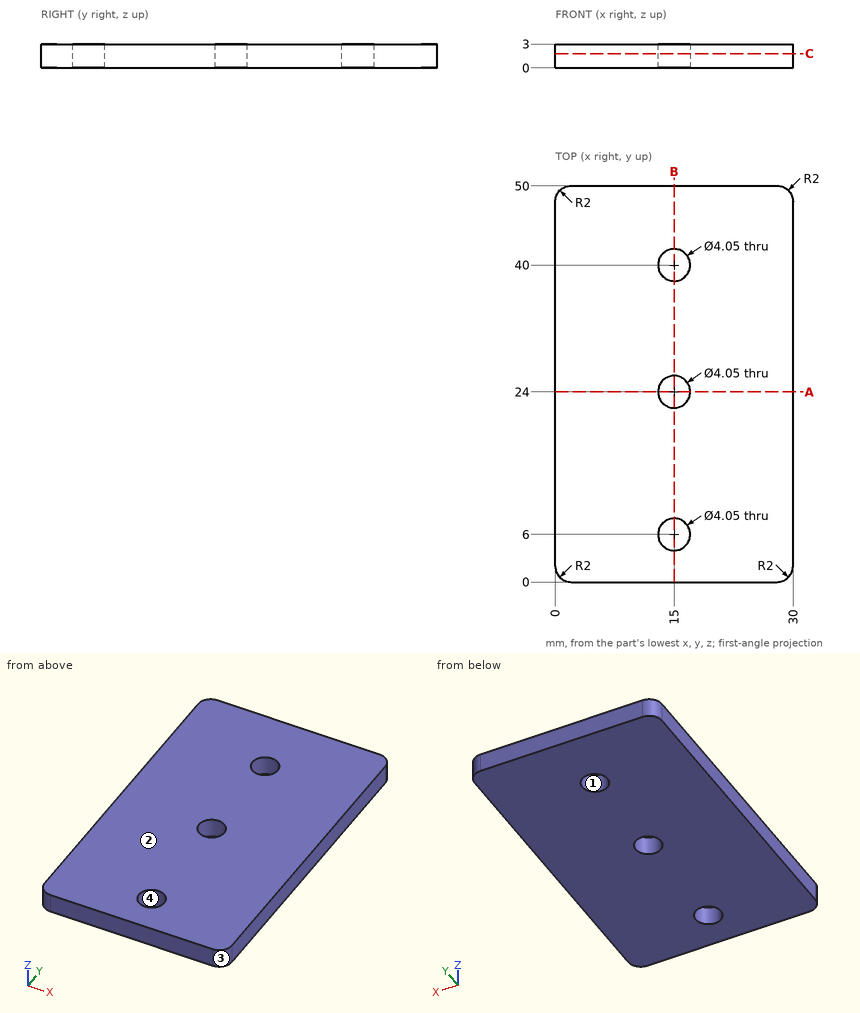
Geometry: see drawing. Coordinates: mm, zero at the bounding-box minimum. Coordinates: 2 decimals unless noted, no trailing zeros. Loops run counter-clockwise (first coordinate to the right, second up) from the corner with the lowest first, then second, coordinate; pieces in that order, holes last. Notation, with made-up numbers: M -9,67.25 L 49,67.25 A17 ccw 49,100.25 Z; hole C 65.5,-10 d6. An arc over 180 degrees is marked long. Answer in a Markdown table with one row per item.
1. Material intervals for line 1 (Y direction, x = 15, z = 2.4) (3 decimals); line 2 (X direction, y = 5, z = 2.2); line 3 (Y direction, x = 28.5, z = 0.9), sorted ascending.
Response:
| item | result |
|---|---|
| line 1 | y = 0 to 3.975, 8.025 to 21.975, 26.025 to 37.975, 42.025 to 50 |
| line 2 | x = 0 to 13.24, 16.76 to 30 |
| line 3 | y = 0.06 to 49.94 |
2. Section C-C, the plane z = 1.8. Output: boundary loops of the cut face in (x, y) (3 decimals), then the cut area to 3 significant figures.
Response:
| item | result |
|---|---|
| outline | M 0,2 A2 ccw 2,0 L 28,0 A2 ccw 30,2 L 30,48 A2 ccw 28,50 L 2,50 A2 ccw 0,48 Z; hole C 15,6 d4.05; hole C 15,24 d4.05; hole C 15,40 d4.05 |
| area | 1,460 mm2 |
3. Section A-A, the plane y = 24. Output: boundary loops of the cut face in (x, z) (3 decimals).
Response:
| item | result |
|---|---|
| outline | M 0,0 L 12.975,0 L 12.975,3 L 0,3 Z; M 17.025,0 L 30,0 L 30,3 L 17.025,3 Z |
4. Section B-B, the plane x = 15. Output: boundary loops of the cut face in (y, z) (3 decimals).
Response:
| item | result |
|---|---|
| outline | M 0,0 L 3.975,0 L 3.975,3 L 0,3 Z; M 8.025,0 L 21.975,0 L 21.975,3 L 8.025,3 Z; M 26.025,0 L 37.975,0 L 37.975,3 L 26.025,3 Z; M 42.025,0 L 50,0 L 50,3 L 42.025,3 Z |
5. Draft query along X for the marked faces 1, 2, 3 and 4. Return one class per face: pulls with the +X half, pulls with the -X half, needs draft (parallel to the pull), parting line crosses it, or undercut.
Response:
| item | result |
|---|---|
| face 1 | undercut |
| face 2 | needs draft |
| face 3 | pulls with the +X half |
| face 4 | undercut |
